Check sheet for the modelled part. Datum: model origin and axes. Units: mm. A direction names the side the tool comes from. Give positions to 0.01 mm unless a question says otherwise; leave off trailing zeros. Order: outer loops, then holes, each group sorted by start corner. A loop starts at its lowest first (then second) coordinate and runs counter-clockwise, first axis right, second up. Notation, with made-up numbers: (-13.75, 63) -> (4.25, 63) arc R18 ccw to (4.25, 82) -> close; hole circle Ø3 at (-26.75, -39). An arc over 180 degrees is marked (long way). Answer in a Markdown table with one row per item. Add a question column.
(1) Set-up check for faces 1 (the face through (38.1, 1, 1)), 2 (the face through (-30.1, 13, 1)), 3 (the face through (-15.748, -44, 1)): record each of +Z, -Z, +X, -X, +Y, -Y from which the full face is reachable in a straight line by a thin tool's end or side.
(2) Cross-section at A-A (z = 2.4). Record the cut outline in (x, y).
(3) Release check for a two-part mould opening along X. For faces 4 (the face through (-34, -25.4, 1)), 5 (the face through (-38.1, -38, 1)), 6 (the face through (15.748, -44, 1)) record: released by +X, released by -X, zero draft, split by the parting line, or undercut.
(4) Thickness scan on L1, parallel to X at y = 33.5, z = 0.2; L2, parallel to Y at x = 19.5, z = 2.15; L3, parallel to Y at x = -17, z = 1.3. Record the ranges inside material, lowest first. Write a range as [from, to].
(5) Go/stop test with flat-tipped pins: pin 1 (1.5 mm diameter, centred on x = 17.5, z = 0.5, fed in from -Y); pin 2 (0.9 mm diameter, centred on y = -4, z = 2, fed in from -X). Record where each tip stops, or that it passes through.
(6) Cross-section at B-B (x = -19.05). Record the cut outline in (y, z).
(7) Cross-section at C-C (y = 39). Record the cut outline in (x, z), then the cut area to 3 significant figures.
```python
from build123d import *

# Parameters (mm, degrees)
PAD_DEPTH = 3


with BuildPart() as part:
    # Sketch → Pad (new body)
    with BuildSketch(Plane.XY):
        with BuildLine():
            ThreePointArc((-29.1, 50.8), (-29.807107, 50.507107), (-30.1, 49.8))
            Line((-30.1, 49.8), (-30.1, -24.4))
            ThreePointArc((-31.1, -25.4), (-30.392893, -25.107107), (-30.1, -24.4))
            Line((-37.1, -25.4), (-31.1, -25.4))
            ThreePointArc((-37.1, -25.4), (-37.807107, -25.692893), (-38.1, -26.4))
            Line((-38.1, -49.8), (-38.1, -26.4))
            ThreePointArc((-38.1, -49.8), (-37.807107, -50.507107), (-37.1, -50.8))
            Line((-37.1, -50.8), (-23.352, -50.8))
            ThreePointArc((-23.352, -50.8), (-22.644893, -50.507107), (-22.352, -49.8))
            Line((-22.352, -38.1), (-22.352, -49.8))
            ThreePointArc((-15.748, -38.1), (-19.05, -34.798), (-22.352, -38.1))
            Line((-15.748, -38.1), (-15.748, -49.8))
            ThreePointArc((-15.748, -49.8), (-15.455107, -50.507107), (-14.748, -50.8))
            Line((-14.748, -50.8), (14.748, -50.8))
            ThreePointArc((14.748, -50.8), (15.455107, -50.507107), (15.748, -49.8))
            Line((15.748, -38.1), (15.748, -49.8))
            ThreePointArc((22.352, -38.1), (19.05, -34.798), (15.748, -38.1))
            Line((22.352, -38.1), (22.352, -49.8))
            ThreePointArc((22.352, -49.8), (22.644893, -50.507107), (23.352, -50.8))
            Line((23.352, -50.8), (37.1, -50.8))
            ThreePointArc((37.1, -50.8), (37.807107, -50.507107), (38.1, -49.8))
            Line((38.1, 49.8), (38.1, -49.8))
            ThreePointArc((38.1, 49.8), (37.807107, 50.507107), (37.1, 50.8))
            Line((-29.1, 50.8), (37.1, 50.8))
        make_face()
    extrude(amount=PAD_DEPTH)


solid = part.part
```
Answer below:
| question | item | result |
|---|---|---|
| 1 | face 1 | +Z, -Z, +X, +Y, -Y |
| 1 | face 2 | +Z, -Z, -X, +Y |
| 1 | face 3 | +Z, -Z, -Y |
| 2 | outline | (-38.1, -49.8) arc R1 ccw to (-37.1, -50.8) -> (-23.35, -50.8) arc R1 ccw to (-22.35, -49.8) -> (-22.35, -38.1) arc R3.3 cw to (-15.75, -38.1) -> (-15.75, -49.8) arc R1 ccw to (-14.75, -50.8) -> (14.75, -50.8) arc R1 ccw to (15.75, -49.8) -> (15.75, -38.1) arc R3.3 cw to (22.35, -38.1) -> (22.35, -49.8) arc R1 ccw to (23.35, -50.8) -> (37.1, -50.8) arc R1 ccw to (38.1, -49.8) -> (38.1, 49.8) arc R1 ccw to (37.1, 50.8) -> (-29.1, 50.8) arc R1 ccw to (-30.1, 49.8) -> (-30.1, -24.4) arc R1 cw to (-31.1, -25.4) -> (-37.1, -25.4) arc R1 ccw to (-38.1, -26.4) -> close |
| 3 | face 4 | zero draft |
| 3 | face 5 | released by -X |
| 3 | face 6 | undercut |
| 4 | L1 | x = [-30.1, 38.1] |
| 4 | L2 | y = [-34.83, 50.8] |
| 4 | L3 | y = [-35.51, 50.8] |
| 5 | pin 1 | stops at y = -35.73 |
| 5 | pin 2 | stops at x = -30.1 |
| 6 | outline | (-34.8, 0) -> (50.8, 0) -> (50.8, 3) -> (-34.8, 3) -> close |
| 7 | outline | (-30.1, 0) -> (38.1, 0) -> (38.1, 3) -> (-30.1, 3) -> close |
| 7 | area | 205 mm² |
